Read the model definition and answer for the solid it produces. Units are mm, in the model's axes. Give positions to 0.01 mm unless a question says otherwise; leave off trailing zeros. Order: outer loops, then holes, each group sorted by start corner. A loop starts at its lowest first (then second) coordinate and runs counter-clockwise, first axis right, second up. Notation, with made-up numbers: (18, 67) - (24, 67) arc R18 cw to (24, 77) - close; hole circle Ø6 at (-7.75, 85). An arc over 180 degrees is marked (long way). Write each question's results on one line, items separated by ' | '.
from build123d import *

# Parameters (mm, degrees)
F0_W     = 15
F0_H     = 39.609302
F0_R     = 6
F1_DEPTH = 3


with BuildPart() as f1:
    # F0 (on Front) → F1 (new body)
    with BuildSketch(Plane.XZ):
        with BuildLine():
            Line((0, 51.938787), (0, 0))
            Line((0, 0), (150, 0))
            Line((150, 0), (300, 0))
            Line((300, 0), (300, 51.938787))
            Line((300, 51.938787), (262.61416, 75.391136))
            Line((262.61416, 75.391136), (236.347529, 75.391136))
            Line((236.347529, 75.391136), (236.347529, 116.513391))
            ThreePointArc((236.347529, 116.513391), (234.946518, 121.618035), (231.13605, 125.292346))
            Line((231.13605, 125.292346), (207.944199, 137.942446))
            Line((207.944199, 137.942446), (170.420438, 137.942446))
            Line((170.420438, 137.942446), (170.420438, 183.440013))
            Line((170.420438, 183.440013), (150, 183.440013))
            Line((150, 183.440013), (129.579562, 183.440013))
            Line((129.579562, 183.440013), (129.579562, 137.942446))
            Line((129.579562, 137.942446), (92.055801, 137.942446))
            Line((92.055801, 137.942446), (68.86395, 125.292346))
            ThreePointArc((68.86395, 125.292346), (65.053482, 121.618035), (63.652471, 116.513391))
            Line((63.652471, 116.513391), (63.652471, 75.391136))
            Line((63.652471, 75.391136), (37.38584, 75.391136))
            Line((37.38584, 75.391136), (0, 51.938787))
        make_face()
        with Locations((40.954411, 38.507754)):
            Rectangle(F0_W, F0_H, mode=Mode.SUBTRACT)
        with Locations((110.85318, 38.507754)):
            Rectangle(F0_W, F0_H, mode=Mode.SUBTRACT)
        with Locations((189.14682, 38.507754)):
            Rectangle(F0_W, F0_H, mode=Mode.SUBTRACT)
        with Locations((259.045589, 38.507754)):
            Rectangle(F0_W, F0_H, mode=Mode.SUBTRACT)
        with Locations((91.120891, 111.901462)):
            Circle(F0_R, mode=Mode.SUBTRACT)
        Polygon((116.900374, 102.314752), (119.052999, 101.753865), (120.974473, 100.633006), (122.52229, 99.035304), (123.581654, 97.079253), (124.073999, 94.909925), (123.962808, 92.688209), (123.256328, 90.578878), (122.006956, 88.738374), (120.307352, 87.303197), (118.283568, 86.379787), (116.085698, 86.036631), (113.876749, 86.299178), (111.820548, 87.147956), (110.069594, 88.520016), (108.753747, 90.313598), (107.970599, 92.39568), (107.77823, 94.611844), (108.190909, 96.797727), (109.178029, 98.791212), (110.66638, 100.444451), (112.545577, 101.634832), (114.676249, 102.274068), align=None, mode=Mode.SUBTRACT)
        with Locations((208.879109, 111.901462)):
            Circle(F0_R, mode=Mode.SUBTRACT)
    extrude(amount=F1_DEPTH)


solid = f1.part
(1) Consider probe 1 along X at (y, z) = (-2.65, 32); probe 2 along Z at (x, y) = (107, -1.25); probe 3 along Z at (x, y) = (261.5, -0.55). Determine where each line is inside the solid, lowest interval first. Write a range as [from, to].
Conclusion:
probe 1: [0, 33.45], [48.45, 103.35], [118.35, 181.65], [196.65, 251.55], [266.55, 300] | probe 2: [0, 18.7], [58.31, 137.94] | probe 3: [0, 18.7], [58.31, 75.39]
(2) Section D-D (y = -0.45) is taken. State how many separate pieces and enclosed holes the cut face has, plus the area to 3 significant figures.
Conclusion:
separate pieces: 1 | enclosed holes: 7 | area: 31,100 mm^2
(3) Each of these flat-tipped pins is pushed along its axis until it touches: pin 1 (0.9 mm diameter, centred on y = -2, z = 105, fed in from -X); pin 2 (0.9 mm diameter, centred on y = -1.5, z = 169.5, fed in from -X); pin 3 (0.9 mm diameter, centred on x = 183, y = -1, fed in from +Z). Where does it stop, or does it pass through?
Conclusion:
pin 1: x = 63.65 | pin 2: x = 129.58 | pin 3: z = 137.94
(4) Section C-C (z = 144) is taken. Give the vertices of the cut face in (x, y), plus the area to 3 significant figures.
Conclusion:
outline: (129.58, -3) - (170.42, -3) - (170.42, 0) - (129.58, 0) - close | area: 123 mm^2
(5) Section B-B (x = 242) is taken. Give the vertices of the cut face in (y, z).
Conclusion:
outline: (-3, 0) - (0, 0) - (0, 75.39) - (-3, 75.39) - close
(6) Section A-A (z = 37.5) is taken. Give the vertices of the cut face in (x, y).
Conclusion:
outline: (0, -3) - (33.45, -3) - (33.45, 0) - (0, 0) - close; (48.45, -3) - (103.35, -3) - (103.35, 0) - (48.45, 0) - close; (118.35, -3) - (181.65, -3) - (181.65, 0) - (118.35, 0) - close; (196.65, -3) - (251.55, -3) - (251.55, 0) - (196.65, 0) - close; (266.55, -3) - (300, -3) - (300, 0) - (266.55, 0) - close
(7) The mould has two halves that part along Z. Classify faces 1 (the face through (204.12, -1.48, 108.25)), 2 (the face through (281.57, -1.48, 63.5)), 3 (the face through (148, 0, 73)): pulls with the +Z half, pulls with the -Z half, needs draft (parallel to the pull), parting line crosses it, or undercut.
Conclusion:
face 1: undercut | face 2: pulls with the +Z half | face 3: needs draft
